Verification items for the finished model (mm, model axes). Coordinates: 2 decimals unless noted, no trailing zeros. Loops run counter-clockwise (first coordinate to the right, second up) from the corner with the lowest first, then second, coordinate; pieces in that order, holes last. Notation, with made-up numbers: (-33, 88.25) - (15, 88.25) arc R20 cw to (15, 121.25) - close; hole circle Ø9 at (11, -36). An arc over 180 degrees is marked (long way). Answer as CSV lines item,"result". Start each with the question number.
1. Material ranges on line 1 (Y direction, x = -6.5, z = 518); line 2 (X direction, y = 3.5, z = 330); line 3 (X direction, y = 9, z = 552), recorded low to high. Write a range as [from, to].
2. Cross-section at A-A (z = 308). Enter the section's corners in (x, y), plus the area to 3 significant figures.
3. Cross-section at B-B (x = 0). State how many separate pieces and enclosed holes the cut face has, plus the area to 3 significant figures.
4. Gauge pin test, flat ends, axial feed: P1, Ø1.6, axis at y = 7, z = 169.5, coming from the +X side; P2, Ø5, axis at x = 0, z = 510, coming from the +Y side; P3, Ø0.6, axis at y = 7, z = 168, coming from the -X side. Record the tip position at first contact, or that the pin passes through.
```python
from build123d import *

# Parameters (mm, degrees)
EXTRUDE_1_DEPTH     = 600
SKETCH_2_R          = 3.25
CUT_EXTRUDE_1_DEPTH = 5.3
SKETCH_3_R          = 2.25
CUT_EXTRUDE_2_DEPTH = 601.125270256


with BuildPart() as part:
    # Model → Бобышка-Вытянуть1 (new body)
    with BuildSketch(Plane.XY):
        with BuildLine():
            Line((6.8, 0), (7.5, 0.7))
            Line((7.5, 0.7), (7.5, 3.6994391))
            Line((7.5, 3.6994391), (4.7998047, 6.3996344))
            Line((4.7998047, 6.3996344), (4.7998047, 8.409149262))
            Line((4.7998047, 8.409149262), (5.20075838, 8.810103152))
            ThreePointArc((5.20075838, 8.810103152), (5.668922208, 9.789261508), (6.648080611, 10.257425237))
            Line((6.648080611, 10.257425237), (7.5, 11.109345046))
            Line((7.5, 11.109345046), (7.5, 12.449454443))
            Line((7.5, 12.449454443), (6.634490912, 13.314965186))
            ThreePointArc((6.634490912, 13.314965186), (5.668922174, 13.781617126), (5.202270193, 14.747185846))
            Line((5.202270193, 14.747185846), (4.949456226, 15))
            Line((4.949456226, 15), (-4.949456226, 15))
            Line((-4.949456226, 15), (-5.202270193, 14.747185846))
            ThreePointArc((-5.202270193, 14.747185846), (-5.668922174, 13.781617126), (-6.634490912, 13.314965186))
            Line((-6.634490912, 13.314965186), (-7.5, 12.449454443))
            Line((-7.5, 12.449454443), (-7.5, 11.109345046))
            Line((-7.5, 11.109345046), (-6.648080611, 10.257425238))
            ThreePointArc((-6.648080611, 10.257425238), (-5.668922208, 9.789261508), (-5.20075838, 8.810103152))
            Line((-5.20075838, 8.810103152), (-4.7998047, 8.409149262))
            Line((-4.7998047, 8.409149262), (-4.7998047, 6.3996344))
            Line((-4.7998047, 6.3996344), (-7.5, 3.6994391))
            Line((-7.5, 3.6994391), (-7.5, 0.7))
            Line((-7.5, 0.7), (-6.8, 0))
            Line((-6.8, 0), (6.8, 0))
        make_face()
    extrude(amount=EXTRUDE_1_DEPTH)

    # Эскиз2 → Вырез-Вытянуть1 (cut)
    with BuildSketch(Plane(origin=(0, 15, 0), x_dir=(1, 0, 0), z_dir=(0, 1, 0))):
        with Locations(Location((0, -30, 0), (0, 0, 180))):
            Circle(SKETCH_2_R)
        with Locations(Location((0, -90, 0), (0, 0, 180))):
            Circle(SKETCH_2_R)
        with Locations(Location((0, -150, 0), (0, 0, 180))):
            Circle(SKETCH_2_R)
        with Locations(Location((0, -210, 0), (0, 0, 180))):
            Circle(SKETCH_2_R)
        with Locations(Location((0, -270, 0), (0, 0, 180))):
            Circle(SKETCH_2_R)
        with Locations(Location((0, -330, 0), (0, 0, 180))):
            Circle(SKETCH_2_R)
        with Locations(Location((0, -390, 0), (0, 0, 180))):
            Circle(SKETCH_2_R)
        with Locations(Location((0, -450, 0), (0, 0, 180))):
            Circle(SKETCH_2_R)
        with Locations(Location((0, -510, 0), (0, 0, 180))):
            Circle(SKETCH_2_R)
        with Locations(Location((0, -570, 0), (0, 0, 180))):
            Circle(SKETCH_2_R)
    extrude(amount=-CUT_EXTRUDE_1_DEPTH, mode=Mode.SUBTRACT)

    # Эскиз3 → Вырез-Вытянуть2 (cut, through all)
    with BuildSketch(Plane(origin=(0, 9.7, 0), x_dir=(1, 0, 0), z_dir=(0, 1, 0))):
        with Locations(Location((0, -30, 0), (0, 0, 180))):
            Circle(SKETCH_3_R)
        with Locations(Location((0, -90, 0), (0, 0, 180))):
            Circle(SKETCH_3_R)
        with Locations(Location((0, -150, 0), (0, 0, 180))):
            Circle(SKETCH_3_R)
        with Locations(Location((0, -210, 0), (0, 0, 180))):
            Circle(SKETCH_3_R)
        with Locations(Location((0, -270, 0), (0, 0, 180))):
            Circle(SKETCH_3_R)
        with Locations(Location((0, -330, 0), (0, 0, 180))):
            Circle(SKETCH_3_R)
        with Locations(Location((0, -390, 0), (0, 0, 180))):
            Circle(SKETCH_3_R)
        with Locations(Location((0, -450, 0), (0, 0, 180))):
            Circle(SKETCH_3_R)
        with Locations(Location((0, -510, 0), (0, 0, 180))):
            Circle(SKETCH_3_R)
        with Locations(Location((0, -570, 0), (0, 0, 180))):
            Circle(SKETCH_3_R)
    extrude(amount=-CUT_EXTRUDE_2_DEPTH, mode=Mode.SUBTRACT)


solid = part.part
```
Values follow:
1,line 1,"y = [0, 4.7], [10.23, 13.34]"
1,line 2,"x = [-7.5, -2.25], [2.25, 7.5]"
1,line 3,"x = [-5.23, 5.23]"
2,outline,"(-7.5, 0.7) - (-6.8, 0) - (6.8, 0) - (7.5, 0.7) - (7.5, 3.7) - (4.8, 6.4) - (4.8, 8.41) - (5.2, 8.81) arc R1.63 cw to (6.65, 10.26) - (7.5, 11.11) - (7.5, 12.45) - (6.63, 13.31) arc R1.63 cw to (5.2, 14.75) - (4.95, 15) - (-4.95, 15) - (-5.2, 14.75) arc R1.63 cw to (-6.63, 13.31) - (-7.5, 12.45) - (-7.5, 11.11) - (-6.65, 10.26) arc R1.63 cw to (-5.2, 8.81) - (-4.8, 8.41) - (-4.8, 6.4) - (-7.5, 3.7) - close"
2,area,"191 mm²"
3,separate pieces,"11"
3,enclosed holes,"0"
3,area,"8,220 mm²"
4,P1,"stops at x = 5"
4,P2,"stops at y = 9.7"
4,P3,"stops at x = -4.8"
